For this review, take the finished solid that the model builds, in its own axes (mm). A direction names the side the tool comes from. Coordinates: 2 decimals unless noted, no trailing zeros. Order: outer loops, then holes, each group sorted by start corner. A loop starts at its lowest first (then second) coordinate and runs counter-clockwise, first axis right, second up. Notation, with made-up numbers: (69, -35.75) - (111, -35.75) arc R30 cw to (111, -5.75) - close; hole circle Ø1 at (22.25, 60). An arc over 180 degrees is marked (long way). One line per item, written item: value. Start each with the question number.
(1) To check wall thickness, follow line 1 along X through (y, z) = (12, 2.3); line 2 along Y through (x, z) = (75, 0.75); line 3 along Y through (x, z) = (10, 1.1). State the ranges of each line that lie inside material, in increasing order.
(2) Consider section D-D on y = 46.15. Write out the cut boundary in (x, z), then the cut area to 3 significant figures.
(3) Consider section C-C on z = 2. Write out the cut boundary in (x, y), then the cut area to 3 significant figures.
(4) Mouldability with a two-part tool opening along X and no side actions: class faces 1 (the flat face through (74, 0, 1)), 2 (the flat face through (150, 12, 1)), 3 (the flat face through (20, 34, 1)), 4 (the cylindrical face through (67.914, 52.597, 1.521)) as released by +X, released by -X, zero draft, split by the parting line, or undercut.
(5) Clearance check with flat-ended pins moving along their axes: pin 1 (0.9 mm diameter, centred on x = 135.5, z = 1.5, fed in from +Y); pin 2 (2.5 mm diameter, centred on x = 67.22, y = 38.37, fed in from -Z); pin 3 (1.5 mm diameter, centred on x = 34, z = 2, fed in from +Y). State where each tip first meets the part, or that it passes through.
(6) For faces 5 (the flat face through (31, 44, 1)), 6 (the flat face through (74, 26, 0)), 7 (the flat face through (119, 44, 1)), list the 3-axis set-ups (+Z, -Z, +X, -X, +Y, -Y) from which the entire face can be reached by the end or side of a thin tool; tool diameter is ignored.
(7) Consider section B-B on y = 12. Write out the cut boundary in (x, z).
(8) Consider section A-A on x = 10. Write out the cut boundary in (y, z).
Autodesk Inventor part; units mm, degrees
ref_plane "YZ Plane" through (0, 0, 0) normal (1, 0, 0) x (0, 1, 0)
ref_plane "XZ Plane" through (0, 0, 0) normal (0, 1, 0) x (-1, 0, 0)
ref_plane "XY Plane" through (0, 0, 0) normal (0, 0, 1) x (1, 0, 0)
sketch "Sketch1" plane through (0, 0, 0) normal (0, 0, 1) x (1, 0, 0)
  line L0 (0, 0) -> (150, 0)
  line L1 (0, 0) -> (0, 24)
  line L2 (0, 24) -> (20, 24)
  circle A0 centre (75, 46.15) radius 8
  line L3 (20, 24) -> (20, 44)
  line L4 (20, 44) -> (56.122, 44)
  line L5 (150, 0) -> (150, 24)
  line L6 (150, 24) -> (130, 24)
  line L7 (130, 24) -> (130, 44)
  line L8 (130, 44) -> (93.878, 44)
  arc A1 (93.878, 44) -> (56.122, 44) centre (75, 46.15) ccw
  dimension "d0" = 150
  dimension "d1" = 24
  dimension "d3" = 16
  dimension "d4" = 20
  dimension "d5" = 38
  dimension "d6" = 75
  dimension "d7" = 22.15
  dimension "d19" = 20
  dimension "d20" = 20
extrude "Extrusion1" add sketch "Sketch1" along normal blind 3
fillet "Fillet1" radius 16 2 edges at (56.122, 44, 1.5) (93.878, 44, 1.5)
sketch "Sketch2" plane through (0, 0, 3) normal (0, 0, 1) x (1, 0, 0)
  circle A0 centre (82.7782, 53.9282) radius 1.5
  circle A1 centre (67.2218, 53.9282) radius 1.5
  circle A2 centre (67.2218, 38.3718) radius 1.5
  circle A3 centre (82.7782, 38.3718) radius 1.5
  circle A4 centre (75, 46.15) radius 8
  circle A5 centre (75, 46.15) radius 11 construction
  line L0 (82.7782, 38.3718) -> (67.2218, 38.3718) construction
  line L1 (67.2218, 38.3718) -> (67.2218, 53.9282) construction
  dimension "d22" = 3
  dimension "d26" = 22
extrude "Extrusion2" cut sketch "Sketch2" against normal up to surface (3 mm away) contours A0 | A1 | A2 | A3
sketch "Sketch3" plane through (0, 0, 3) normal (0, 0, 1) x (1, 0, 0)
  line L0 (0, 0) -> (150, 0)
  line L1 (150, 0) -> (150, 24)
  line L2 (0, 24) -> (0, 0)
  point P0 (10, 12)
  point P1 (140, 12)
  dimension "d27" = 10
  dimension "d28" = 10
  dimension "d29" = 12
hole "Hole1" at (10, 12, 3) at (140, 12, 3) direction (0, 0, -1) diameter 5 end through all
properties part number "ZAxisNutMountMetal" material "Steel, Alloy"
Geometry check:
1. line 1: x = 0 to 7.5, 12.5 to 137.5, 142.5 to 150
1. line 2: y = 0 to 38.15, 54.15 to 65.15
1. line 3: y = 0 to 9.5, 14.5 to 24
2. outline: (50.87, 0) - (67, 0) - (67, 3) - (50.87, 3) - close; (83, 0) - (99.13, 0) - (99.13, 3) - (83, 3) - close
2. area: 96.8 mm^2
3. outline: (0, 0) - (150, 0) - (150, 24) - (130, 24) - (130, 44) - (107.14, 44) arc R16 cw to (92.45, 53.67) arc R19 ccw to (57.55, 53.67) arc R16 cw to (42.86, 44) - (20, 44) - (20, 24) - (0, 24) - close; hole circle Ø5 at (10, 12); hole circle Ø3 at (67.22, 38.37); hole circle Ø3 at (67.22, 53.93); hole circle Ø16 at (75, 46.15); hole circle Ø3 at (82.78, 38.37); hole circle Ø3 at (82.78, 53.93); hole circle Ø5 at (140, 12)
3. area: 6,240 mm^2
4. face 1: zero draft
4. face 2: released by +X
4. face 3: released by -X
4. face 4: undercut
5. pin 1: stops at y = 24
5. pin 2: passes through
5. pin 3: stops at y = 44
6. face 5: +Z, -Z, -X, +Y
6. face 6: -Z, +X, -X, +Y, -Y
6. face 7: +Z, -Z, +X, +Y
7. outline: (0, 0) - (7.5, 0) - (7.5, 3) - (0, 3) - close; (12.5, 0) - (137.5, 0) - (137.5, 3) - (12.5, 3) - close; (142.5, 0) - (150, 0) - (150, 3) - (142.5, 3) - close
8. outline: (0, 0) - (9.5, 0) - (9.5, 3) - (0, 3) - close; (14.5, 0) - (24, 0) - (24, 3) - (14.5, 3) - close
